```python
from build123d import *

# Parameters (mm, degrees)
BOSS_EXTRUDE3_DEPTH = 5


with BuildPart() as part:
    # Sketch1 → Boss-Extrude3 (new body)
    with BuildSketch(Plane.XY):
        with BuildLine():
            Line((-27.5, 0), (-24.5, 0))
            ThreePointArc((-24.5, 0), (-23.822061062, 5.723583386), (-21.825762712, 11.130412483))
            ThreePointArc((-21.825762712, 11.130412483), (-21.418354885, 12.233846993), (-21.28, 13.401925235))
            Line((-21.28, 13.401925235), (-21.28, 14.540127049))
            ThreePointArc((-21.28, 14.540127049), (-21.053037703, 16.029459479), (-20.392755565, 17.383582985))
            ThreePointArc((-20.392755565, 17.383582985), (-18.722329772, 19.255294032), (-16.644357741, 20.660874629))
            ThreePointArc((-16.644357741, 20.660874629), (0, 24.5), (16.644357741, 20.660874629))
            ThreePointArc((16.644357741, 20.660874629), (18.722329772, 19.255294032), (20.392755565, 17.383582985))
            ThreePointArc((20.392755565, 17.383582985), (21.053037703, 16.029459479), (21.28, 14.540127049))
            Line((21.28, 14.540127049), (21.28, 13.401925235))
            ThreePointArc((21.28, 13.401925235), (21.418354885, 12.233846993), (21.825762712, 11.130412483))
            ThreePointArc((21.825762712, 11.130412483), (23.822061062, 5.723583386), (24.5, 0))
            Line((24.5, 0), (27.5, 0))
            ThreePointArc((27.5, 0), (26.682859667, 6.653946198), (24.28, 12.9124591))
            Line((24.28, 12.9124591), (24.28, 19.537578604))
            ThreePointArc((24.28, 19.537578604), (0, 27.5), (-24.28, 19.537578604))
            Line((-24.28, 19.537578604), (-24.28, 12.9124591))
            ThreePointArc((-24.28, 12.9124591), (-26.682859667, 6.653946198), (-27.5, 0))
        make_face()
    extrude(amount=BOSS_EXTRUDE3_DEPTH)


solid = part.part
```
The model under review builds one solid part; all positions refer to its coordinate system, in mm. A direction names the side the tool comes from. Coordinates: 2 decimals unless noted, no trailing zeros. Write each loop counter-clockwise with the first axis right and the second up, starting at its lowest first coordinate (ties: lowest second). Pieces come first, ordered by that corner, then holes. Notation, with made-up numbers: (84, 89) - (122, 89) arc R28 ccw to (122, 126) - close; hole circle Ø11 at (36, -38). An arc over 180 degrees is marked (long way). Write item = value, one per line.
(1) For P1, Ø0.6, axis at y = 14, z = 2, coming from the -X side; P2, Ø2.5, axis at y = 16, z = 2, coming from the +X side; P3, Ø1.5, axis at x = 0, z = 3.5, coming from the +Y side, all flat-tipped, find the tip position at first contact; note any pin that passes through.
Result sheet:
P1 = -24.28
P2 = 24.28
P3 = 27.5
(2) Consider section B-B, the plane y = 10.25. Give the boundary of the cut face in (x, z), then the cut area to 3 significant figures.
Result sheet:
outline = (-25.52, 0) - (-22.25, 0) - (-22.25, 5) - (-25.52, 5) - close; (22.25, 0) - (25.52, 0) - (25.52, 5) - (22.25, 5) - close
area = 32.7 mm^2
(3) Consider section C-C, the plane y = 21.5. Give the boundary of the cut face in (x, z), then the cut area to 3 significant figures.
Result sheet:
outline = (-21.35, 0) - (-14.8, 0) - (-14.8, 5) - (-21.35, 5) - close; (14.8, 0) - (21.35, 0) - (21.35, 5) - (14.8, 5) - close
area = 65.6 mm^2
(4) Mouldability with a two-part tool opening along X and no side actions: class faces 6 (the face through (23.803, 5.802, 2.465)), 7 (the face through (-26, 0, 2)), 8 (the face through (-26.66, 6.75, 2.46)), 9 (the face through (-21.06, 16.01, 2.46)) as pulls with the +X half, pulls with the -X half, needs draft (parallel to the pull), parting line crosses it, or undercut.
Result sheet:
face_6 = undercut
face_7 = needs draft
face_8 = pulls with the -X half
face_9 = undercut
(5) Consider section A-A, the plane z = 3.4. Give the boundary of the cut face in (x, y).
Result sheet:
outline = (-27.5, 0) - (-24.5, 0) arc R24.5 cw to (-21.83, 11.13) arc R5 ccw to (-21.28, 13.4) - (-21.28, 14.54) arc R5 cw to (-20.39, 17.38) arc R10.16 cw to (-16.64, 20.66) arc R38 cw to (16.64, 20.66) arc R10.16 cw to (20.39, 17.38) arc R5 cw to (21.28, 14.54) - (21.28, 13.4) arc R5 ccw to (21.83, 11.13) arc R24.5 cw to (24.5, 0) - (27.5, 0) arc R27.5 ccw to (24.28, 12.91) - (24.28, 19.54) arc R41 ccw to (-24.28, 19.54) - (-24.28, 12.91) arc R27.5 ccw to start
(6) Consider section D-D, the plane x = 18. Give the boundary of the cut face in (y, z).
Result sheet:
outline = (19.83, 0) - (23.34, 0) - (23.34, 5) - (19.83, 5) - close
(7) For line 1 (X direction, y = 14.75, z = 2.95); line 2 (X direction, y = 11.5, z = 3.8); line 3 (Y direction, x = 13.5, z = 1.3), list the stretches that pass through material, from the lowest coordinate up. Write a range as [from, to].
Result sheet:
line_1 = [-24.28, -21.28], [21.28, 24.28]
line_2 = [-24.98, -21.66], [21.66, 24.98]
line_3 = [22.02, 25.21]
(8) Machinability: for faces 1 (the face through (24.28, 16, 2)), 2 (the face through (0, 25, 0)), 3 (the face through (21.415, 12.25, 2.465)), 4 (the face through (-24.28, 16, 2)), 5 (the face through (0, 25, 5)), which of the approach directions +Z, -Z, +X, -X, +Y, -Y give a long, thin tool a straight path to every point of the face, cutting with its end or side? Answer none if there is none.
Result sheet:
face_1 = +Z, -Z, +X, +Y
face_2 = -Z, +X, -X, +Y, -Y
face_3 = +Z, -Z, -Y
face_4 = +Z, -Z, -X, +Y
face_5 = +Z, +X, -X, +Y, -Y
